Can you work these out from the model? Positions are in its coordinate system, mm. A direction names the side the tool comes from. Give positions to 0.01 mm unless a question says otherwise; leave off trailing zeros. Loops run counter-clockwise (first coordinate to the right, second up) from the corner with the lowest first, then second, coordinate; pieces in that order, holes last. Notation, with made-up numbers: (12, 73.5) -> (19, 73.5) arc R29 cw to (19, 96.5) -> close; hole circle Ø3 at (79, 36). An arc over 180 degrees is marked (long way). Use CSV: the item, a comma, the result in double quotes.
from build123d import *

# Parameters (mm, degrees)
F0_W     = 60.269747
F0_H     = 50.542671
F1_DEPTH = 36.65792
F3_DEPTH = 25.4


with BuildPart() as f1:
    # F0 (on Top) → F1 (new body)
    with BuildSketch(Plane.XY):
        with Locations((6.293992, -1.144362)):
            Rectangle(F0_W, F0_H)
    extrude(amount=F1_DEPTH)

    # F2 (on face) → F3 (cut)
    with BuildSketch(Plane.XY.offset(36.65792)):
        Polygon((0, 0), (-23.840882, -26.415698), (0, -26.415698), align=None)
    extrude(amount=-F3_DEPTH, mode=Mode.SUBTRACT)


solid = f1.part
(1) Which directions (+Z, -Z, +X, -X, +Y, -Y) give clear straight access to the entire face, cutting with the end or side of a thin tool? Please do faces 1 (the face through (-11.75, -13.02, 24.14)), 2 (the face through (6, 24.127, 18)).
Answer sheet:
face 1,"+Z, -Y"
face 2,"+Z, -Z, +X, -X, +Y"
(2) We'd pull the mould along X, two halves only. Please class faces 3 (the face through (0, -13, 24)), 4 (the face through (36.429, -1, 18)), 5 (the face through (6, -1, 36.658)): released by +X, released by -X, zero draft, split by the parting line, or undercut.
Answer sheet:
face 3,"undercut"
face 4,"released by +X"
face 5,"zero draft"
(3) Will this pin go through, and if not, where does the flat tip stop? pin 1 Ø3 at (x, z) = (-2.5, 15) entering from -Y.
Answer sheet:
pin 1,"stops at y = -4.43"
(4) If I drill on L1, parallel to X at y = -19, z = 20.5; L2, parallel to X at y = -13, z = 33; L3, parallel to Y at x = -13, z = 16.5, over which ranges is the centre line in solid material (lowest first)? Write a range as from..to.
Answer sheet:
L1,"x = -23.84..-17.15, 0..36.43"
L2,"x = -23.84..-11.73, 0..36.43"
L3,"y = -14.4..24.13"
(5) If we section it at C-C, the plane z = 28.5: Write out the boundary of the cut face in (x, y), then the cut area to 3 significant figures.
Answer sheet:
outline,"(-23.84, -26.42) -> (0, 0) -> (0, -26.42) -> (36.43, -26.42) -> (36.43, 24.13) -> (-23.84, 24.13) -> close"
area,"2,730 mm2"
(6) If we section it at B-B, the plane y = -19.5: Write out the boundary of the cut face in (x, z).
Answer sheet:
outline,"(-23.84, 0) -> (36.43, 0) -> (36.43, 36.66) -> (0, 36.66) -> (0, 11.26) -> (-17.6, 11.26) -> (-17.6, 36.66) -> (-23.84, 36.66) -> close"
(7) If we section it at A-A, the plane x = -10: Write out the boundary of the cut face in (y, z).
Answer sheet:
outline,"(-26.42, 0) -> (24.13, 0) -> (24.13, 36.66) -> (-11.08, 36.66) -> (-11.08, 11.26) -> (-26.42, 11.26) -> close"
